Autodesk Inventor part; units mm, degrees
ref_plane "YZ Plane" through (0, 0, 0) normal (1, 0, 0) x (0, 1, 0)
ref_plane "XZ Plane" through (0, 0, 0) normal (0, 1, 0) x (-1, 0, 0)
ref_plane "XY Plane" through (0, 0, 0) normal (0, 0, 1) x (1, 0, 0)
sketch "スケッチ1" plane through (0, 0, 0) normal (0, 0, 1) x (1, 0, 0)
  point P0 (0, 0)
sketch "スケッチ2" plane through (0, 0, 0) normal (0, 0, 1) x (1, 0, 0)
  line L0 (0, 0) -> (15, 0)
  line L1 (15, 0) -> (15, 30)
  line L2 (15, 30) -> (0, 30)
  line L3 (0, 30) -> (0, 0)
  dimension "d0" = 15
  dimension "d1" = 30
extrude "押し出し1" add sketch "スケッチ2" along normal blind 770
sketch "スケッチ3" plane through (0, 0, 770) normal (0, 0, 1) x (1, 0, 0)
  line L0 (1, 1) -> (14, 1)
  line L1 (14, 1) -> (14, 29)
  line L2 (14, 29) -> (1, 29)
  line L3 (1, 29) -> (1, 1)
  line L4 (0, 30) -> (0, 0)
  line L5 (0, 0) -> (15, 0)
  dimension "d4" = 13
  dimension "d5" = 28
  dimension "d6" = 1
  dimension "d7" = 1
extrude "押し出し2" cut sketch "スケッチ3" against normal blind 770
sketch "スケッチ4" plane through (0, 30, 770) normal (0, 1, 0) x (1, 0, 0)
  circle A0 centre (7.5, 123) radius 1.65
  line L0 (0, 770) -> (0, 0)
  line L1 (15, 0) -> (0, 0)
  circle A1 centre (7.5, 133) radius 1.65
  circle A2 centre (7.5, 143) radius 1.65
  dimension "d10" = 3.3
  dimension "d11" = 7.5
  dimension "d12" = 123
  dimension "d13" = 3.3
  dimension "d14" = 3.3
  dimension "d15" = 10
  dimension "d16" = 7.5
  dimension "d17" = 10
  dimension "d18" = 7.5
hole "穴1" at (7.5, 30, 647) at (7.5, 30, 637) at (7.5, 30, 627) direction (0, -1, 0) diameter 3.4 depth 30
equation "\"BendRadius\" = Thickness"
equation "\"BendReliefWidth\" = Thickness"
equation "\"BendReliefDepth\" = 0.5 * Thickness"
equation "\"CornerReliefSize\" = 4 * Thickness"
equation "\"MinimumRemnant\" = 2 * Thickness"
equation "\"TransitionRadius\" = BendRadius"
equation "\"JacobiRadiusSize\" = BendRadius"
equation "\"GapSize\" = Thickness"
properties part number "オムニ_角柱1_N"
The model under review builds one solid part; all positions refer to its coordinate system, in mm. A direction names the side the tool comes from. Give positions to 0.01 mm unless a question says otherwise; leave off trailing zeros. Write each loop counter-clockwise with the first axis right and the second up, starting at its lowest first coordinate (ties: lowest second). Pieces come first, ordered by that corner, then holes. Notation, with made-up numbers: M 43,67 L 52,67 A21 cw 52,76 Z; hole C 31,61 d7. An arc over 180 degrees is marked long. Write item = value, one per line. Start each with the question number.
Q1. Machinability: for faces 5 (the face through (7, 1, 390)), 6 (the face through (7, 0, 380)), which of the approach directions +Z, -Z, +X, -X, +Y, -Y give a long, thin tool a straight path to every point of the face, cutting with its end or side? Answer none if there is none.
Q2. We need section A-A (y = 10.75). State the section outline as (x, z) points, plus the area to 3 significant figures.
Q3. Clearance check with flat-ended pins moving along their axes: pin 1 (4.5 mm diameter, centred on x = 7.5, z = 647, fed in from +Y); pin 2 (2 mm diameter, centred on x = 7.5, z = 637, fed in from +Y). State where each tip first meets the part, or that it passes through.
Q4. We need section B-B (z = 169.5). State the section outline as (x, y) points, plus the area to 3 significant figures.
Q5. For line 1 (Z direction, x = 7.5, y = 0.6); line 2 (Y direction, x = 13.5, z = 380.5); line 3 (X direction, y = 0.55, z = 637), list the stretches that pass through material, from the lowest coordinate up.
Q6. Mouldability with a two-part tool opening along Y and no side actions: class faces 1 (the face through (8, 29, 390)), 2 (the face through (0.8, 16.2, 0)), 3 (the face through (14, 15, 390)), 4 (the face through (8, 30, 380)) as released by +Y, released by -Y, zero draft, split by the parting line, or undercut.
Result set:
q1.face_5 = +Z, -Z
q1.face_6 = +Z, -Z, +X, -X, -Y
q2.outline = M 0,0 L 1,0 L 1,770 L 0,770 Z; M 14,0 L 15,0 L 15,770 L 14,770 Z
q2.area = 1,540 mm2
q3.pin_1 = 30
q3.pin_2 = through
q4.outline = M 0,0 L 15,0 L 15,30 L 0,30 Z; hole M 1,1 L 14,1 L 14,29 L 1,29 Z
q4.area = 86.0 mm2
q5.line_1 = 0 to 625.3, 628.7 to 635.3, 638.7 to 645.3, 648.7 to 770
q5.line_2 = 0 to 1, 29 to 30
q5.line_3 = 0 to 5.8, 9.2 to 15
q6.face_1 = undercut
q6.face_2 = zero draft
q6.face_3 = undercut
q6.face_4 = released by +Y
